For this review, take the finished solid that the model builds, in its own axes (mm). A direction names the side the tool comes from. Coordinates: 2 decimals unless noted, no trailing zeros. Order: outer loops, then holes, each group sorted by start corner. A loop starts at its lowest first (then second) coordinate and runs counter-clockwise, first axis right, second up.
from build123d import *

# Parameters (mm, degrees)
F0_W     = 40
F0_H     = 5
F0_R     = 2
F1_DEPTH = 10
F2_R     = 1
F3_DEPTH = 10
F4_SIZE  = 5


with BuildPart() as f1:
    # F0 (on Top) → F1 (new body)
    with BuildSketch(Plane.XY):
        with Locations((0, -9.5)):
            Rectangle(F0_W, F0_H)
        with BuildLine():
            Line((-9.814244, 5.368419), (-20, -7))
            Line((-20, -7), (20, -7))
            Line((20, -7), (9.814244, 5.368419))
            ThreePointArc((9.814244, 5.368419), (5.426116, 8.783949), (0, 10))
            ThreePointArc((0, 10), (-5.426116, 8.783949), (-9.814244, 5.368419))
        make_face()
        Circle(F0_R, mode=Mode.SUBTRACT)
    extrude(amount=F1_DEPTH)

    # F2 (on face) → F3 (cut)
    with BuildSketch(Plane.XZ.offset(12)):
        with Locations((-14, 4)):
            Circle(F2_R)
        with Locations((14, 4)):
            Circle(F2_R)
    extrude(amount=-F3_DEPTH, mode=Mode.SUBTRACT)

    # F4
    f4_edges = [f1.edges().sort_by_distance(p)[0] for p in [
        (14.907122, -0.815791, 10),
    ]]
    chamfer(f4_edges, length=F4_SIZE)


solid = f1.part
1. Take a section at D-D, the plane z = 4. Give the boundary of the cut face in (x, y), plus the area to 3 significant figures.
Answer below:
outline: (-20, -12) - (-15, -12) - (-15, -2) - (-13, -2) - (-13, -12) - (13, -12) - (13, -2) - (15, -2) - (15, -12) - (20, -12) - (20, -7) - (9.81, 5.37) arc R12.71 ccw to (0, 10) arc R12.71 ccw to (-9.81, 5.37) - (-20, -7) - close; hole circle Ø4 at (0, 0)
area: 579 mm2
2. The part is to be moulded in two halves that separate along Y. For faces 3 (the face through (14.978, -0.902, 2.465)), 4 (the face through (0, -2, 5)), 5 (the face through (14, -2, 4)), 6 (the face through (0, -5, 10)), say which applies: +Y half, -Y half, draft (parallel to the pull), parting line (faces both ways), or undercut.
Answer below:
face 3: +Y half
face 4: undercut
face 5: -Y half
face 6: draft
3. Take a section at A-A, the plane z = 1.5. Give the boundary of the cut face in (x, y), plus the area to 3 significant figures.
Answer below:
outline: (-20, -12) - (20, -12) - (20, -7) - (9.81, 5.37) arc R12.71 ccw to (0, 10) arc R12.71 ccw to (-9.81, 5.37) - (-20, -7) - close; hole circle Ø4 at (0, 0)
area: 619 mm2
4. Clearance check with flat-ended pins moving along their axes: pin 1 Ø1.6 at (x, z) = (-14, 4) entering from -Y; pin 2 Ø3 at (x, z) = (14, 4) entering from +Y; pin 3 Ø1.5 at (x, y) = (6, 7) entering from +Z. State where each tip first meets the part, or that it passes through.
Answer below:
pin 1: stops at y = -2
pin 2: stops at y = 2.11
pin 3: stops at z = 7.05
5. Machinability: for faces 1 (the face through (0, -3, 0)), 2 (the face through (-14, -2, 4)), which of the approach directions +Z, -Z, +X, -X, +Y, -Y give a long, thin tool a straight path to every point of the face, cutting with its end or side? Answer none if there is none.
Answer below:
face 1: -Z, +X, -X, +Y, -Y
face 2: -Y
6. To check wall thickness, follow L1, parallel to Y at x = 0, z = 1.75; L2, parallel to Z at x = -14, y = -9.5. State the ranges of each line that lie inside material, in increasing order.
Answer below:
L1: y = -12 to -2, 2 to 10
L2: z = 0 to 3, 5 to 10
7. Take a section at B-B, the plane y = -6. Give the boundary of the cut face in (x, z).
Answer below:
outline: (-19.18, 0) - (19.18, 0) - (19.18, 5) - (12.7, 10) - (-12.7, 10) - (-19.18, 5) - close; hole circle Ø2 at (-14, 4); hole circle Ø2 at (14, 4)
8. Take a section at C-C, the plane y = 0. Give the boundary of the cut face in (x, z), plus the area to 3 significant figures.
Answer below:
outline: (-14.24, 0) - (-2, 0) - (-2, 10) - (-7.76, 10) - (-14.24, 5) - close; (2, 0) - (14.24, 0) - (14.24, 5) - (7.76, 10) - (2, 10) - close
area: 212 mm2
